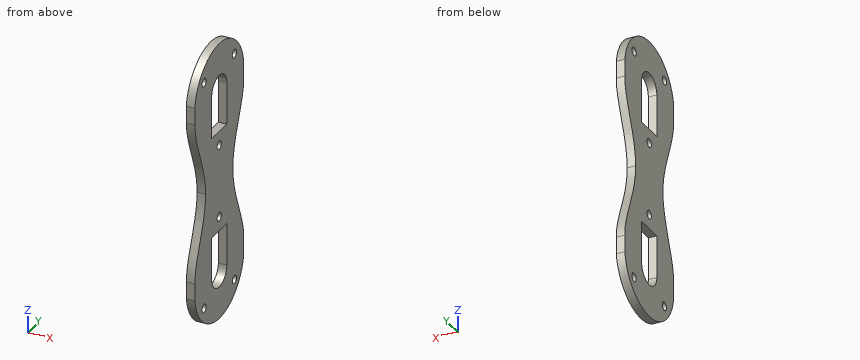
```python
from build123d import *

# Parameters (mm, degrees)
SCHIZZO1_R                   = 1
ESTRUSIONE_ESTRUSIONE1_DEPTH = 2


with BuildPart() as part:
    # Schizzo1 → Estrusione-Estrusione1 (new body)
    with BuildSketch(Plane(origin=(0, 0, 0), x_dir=(0, 0, -1), z_dir=(1, 0, 0))):
        with BuildLine():
            Line((-2.501010101, -11.3), (1.498989899, -11.3))
            ThreePointArc((1.498989899, -11.3), (11.398989899, 0), (1.498989899, 11.3))
            Line((1.498989899, 11.3), (-2.501010101, 11.3))
            add(Edge.make_bspline(
                [(-2.501010101, 11.3), (-7.839898951, 11.429610053), (-14.35178918, 6.216652626), (-21.601010101, 6.3)],
                knots=[0, 0, 0, 0, 1, 1, 1, 1], degree=3))
            add(Edge.make_bspline(
                [(-40.701010101, 11.3), (-35.362121251, 11.429610053), (-28.850231022, 6.216652626), (-21.601010101, 6.3)],
                knots=[0, 0, 0, 0, 1, 1, 1, 1], degree=3))
            Line((-40.701010101, 11.3), (-44.701010101, 11.3))
            ThreePointArc((-44.701010101, 11.3), (-54.601010101, 0), (-44.701010101, -11.3))
            Line((-44.701010101, -11.3), (-40.701010101, -11.3))
            add(Edge.make_bspline(
                [(-40.701010101, -11.3), (-34.455779635, -11.063584615), (-28.769360616, -6.33994929), (-21.601010101, -6.3)],
                knots=[0, 0, 0, 0, 1, 1, 1, 1], degree=3))
            add(Edge.make_bspline(
                [(-2.501010101, -11.3), (-8.746240567, -11.063584615), (-14.432659586, -6.33994929), (-21.601010101, -6.3)],
                knots=[0, 0, 0, 0, 1, 1, 1, 1], degree=3))
        make_face()
        with Locations((-48.702020202, 7)):
            Circle(SCHIZZO1_R, mode=Mode.SUBTRACT)
        with Locations((-48.702020202, -7)):
            Circle(SCHIZZO1_R, mode=Mode.SUBTRACT)
        with Locations((-30.202020202, 0)):
            Circle(SCHIZZO1_R, mode=Mode.SUBTRACT)
        with Locations((-13, 0)):
            Circle(SCHIZZO1_R, mode=Mode.SUBTRACT)
        with Locations((5.5, 7)):
            Circle(SCHIZZO1_R, mode=Mode.SUBTRACT)
        with Locations((5.5, -7)):
            Circle(SCHIZZO1_R, mode=Mode.SUBTRACT)
        with BuildLine():
            Line((-9.676010101, 3.5), (0.323989899, 3.5))
            ThreePointArc((0.323989899, 3.5), (3.823989899, 0), (0.323989899, -3.5))
            Line((0.323989899, -3.5), (-9.676010101, -3.5))
            Line((-9.676010101, -3.5), (-9.676010101, 3.5))
        make_face(mode=Mode.SUBTRACT)
        with BuildLine():
            Line((-33.526010101, -3.5), (-43.526010101, -3.5))
            ThreePointArc((-43.526010101, -3.5), (-47.026010101, 0), (-43.526010101, 3.5))
            Line((-43.526010101, 3.5), (-33.526010101, 3.5))
            Line((-33.526010101, 3.5), (-33.526010101, -3.5))
        make_face(mode=Mode.SUBTRACT)
    extrude(amount=ESTRUSIONE_ESTRUSIONE1_DEPTH)


solid = part.part
```
The listing builds one solid part. Answer for the finished solid, in the listing's coordinates (mm). Give positions to 0.01 mm unless a question says otherwise; leave off trailing zeros. Order: outer loops, then holes, each group sorted by start corner. A loop starts at its lowest first (then second) coordinate and runs counter-clockwise, first axis right, second up. Notation, with made-up numbers: (88, 45) -> (103, 45) arc R8 ccw to (103, 53) -> close; hole circle Ø5 at (8.5, 5). An arc over 180 degrees is marked (long way). Answer as a JSON object with one key per item and string values. Group by question number.
Item 1: The part is cut by section C-C on z = -5.5. Write down the section's boundary in (x, y).
Item 2: The part is cut by section A-A on y = 0. Write down the section's boundary in (x, z), and give its area (3 significant figures).
Item 3: The part is cut by section B-B on x = 1.05. Give the number of separate pieces and of enclosed holes in the cut face, and give its area (3 significant figures).
Item 4: Consider L1, parallel to Y at x = 0.9, z = -5.5; L2, parallel to Y at x = 1.4, z = 40.5; L3, parallel to Z at x = 0.8, y = 1.5. Determine where each line is inside the solid, lowest interval first. Write a range as from..to.
Item 5: Flat-ended cylindrical pins translate along their axes: pin 1 (0.6 mm diameter, centred on x = 0.5, z = 1.5, fed in from +Y); pin 2 (0.6 mm diameter, centred on x = 1.5, y = 0.5, fed in from -Z); pin 3 (0.6 mm diameter, centred on x = 0.5, z = 40, fed in from -Y). Find the tip coordinate at first contact, or state that the pin passes through.
Result set:
{
 "1": {"outline": "(0, -9.98) -> (2, -9.98) -> (2, -8) -> (0, -8) -> close; (0, -6) -> (2, -6) -> (2, 6) -> (0, 6) -> close; (0, 8) -> (2, 8) -> (2, 9.98) -> (0, 9.98) -> close"},
 "2": {"outline": "(0, -11.4) -> (2, -11.4) -> (2, -3.82) -> (0, -3.82) -> close; (0, 9.68) -> (2, 9.68) -> (2, 12) -> (0, 12) -> close; (0, 14) -> (2, 14) -> (2, 29.2) -> (0, 29.2) -> close; (0, 31.2) -> (2, 31.2) -> (2, 33.53) -> (0, 33.53) -> close; (0, 47.03) -> (2, 47.03) -> (2, 54.6) -> (0, 54.6) -> close", "area": "70.0 mm²"},
 "3": {"separate pieces": "1", "enclosed holes": "8", "area": "986 mm²"},
 "4": {"L1": "-9.98..-8, -6..6, 8..9.98", "L2": "-11.29..-3.5, 3.5..11.3", "L3": "-11.3..-3.49, 9.68..33.53, 46.69..54.5"},
 "5": {"pin 1": "y = 11.3", "pin 2": "z = -11.4", "pin 3": "y = -11.28"}
}
